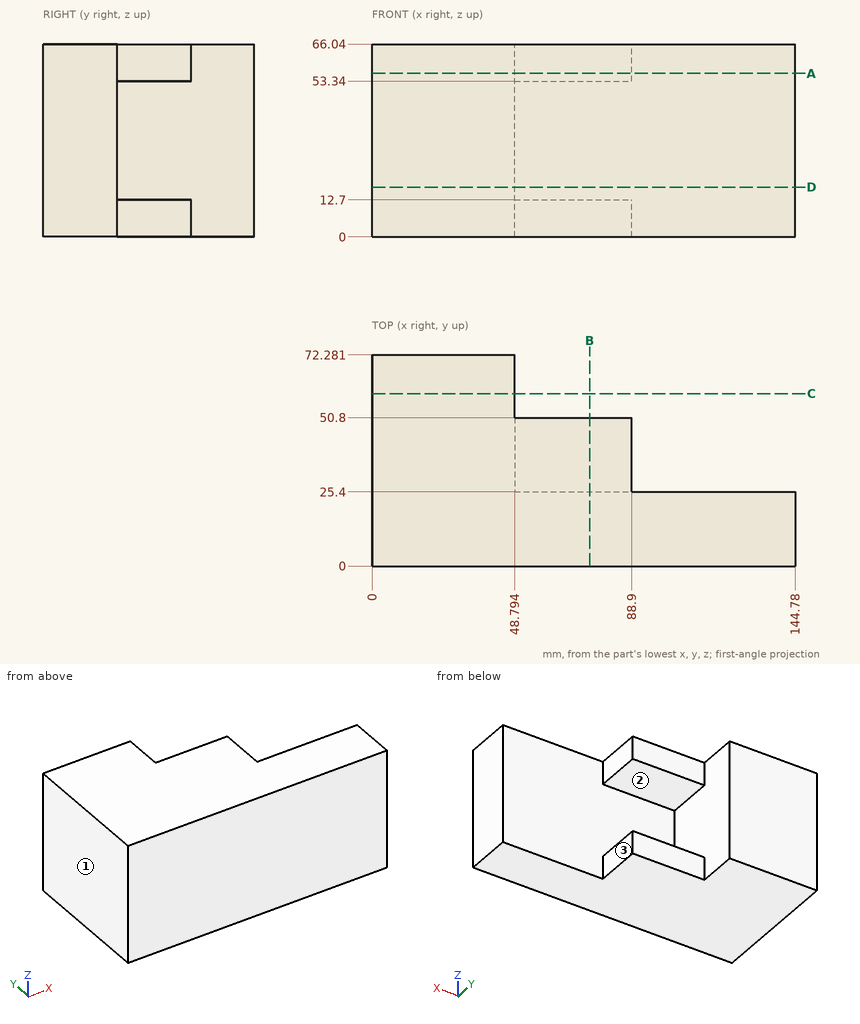
Source: three-view drawing plus pictorial views. Frame: mm from the lowest corner of the part. A direction names the side the tool comes from. Round coordinates to 2 decimals unless told otherwise and drop trailing zeros. Loops run counter-clockwise (first coordinate to the right, second up) from the corner with the lowest first, then second, coordinate; pieces in that order, holes last.
1. Contact query for flat-ended pins moving along their axis: pin 1 (14 mm diameter, centred on x = 76.5, z = 57.5, fed in from +Y); pin 2 (10 mm diameter, centred on y = 36, z = 57, fed in from +X); pin 3 (2 mm diameter, centred on x = 29, y = 35.5, fed in from -Z); pin 4 (4 mm diameter, centred on x = 120, z = 56.5, fed in from +Y). Output: stop coordinate, or through.
2. Access query for the marked faces 1, 2 and 3. Directions: +Z, -Z, +X, -X, +Y, -Y. A direction counts if a zero-diameter tool reaches every point of the face in a straight line with its end or side. Return the directions, or none.
3. Section query A-A on z = 56. Output: boundary loops of the cut face in (x, y).
4. Section query C-C on y = 59. Output: boundary loops of the cut face in (x, z).
5. Ray query, L1, parallel to Z at x = 51, y = 38; L2, parallel to X at y = 44, z = 61; L3, parallel to X at y = 47.5, z = 15.5. Return the intervals inside material, ascending.
6. Section query B-B on x = 74.5. Output: boundary loops of the cut face in (y, z), and give its area (3 significant figures).
7. Section query D-D on z = 17. Output: boundary loops of the cut face in (x, y), and give its area (4 significant figures).
Answers below:
1. pin 1: stops at y = 50.8
1. pin 2: stops at x = 88.9
1. pin 3: stops at z = 0
1. pin 4: stops at y = 25.4
2. face 1: +Z, -Z, -X, +Y, -Y
2. face 2: +X, +Y
2. face 3: +Z, -Z, +X, +Y
3. outline: (0, 0) - (144.78, 0) - (144.78, 25.4) - (88.9, 25.4) - (88.9, 50.8) - (48.79, 50.8) - (48.79, 72.28) - (0, 72.28) - close
4. outline: (0, 0) - (48.79, 0) - (48.79, 66.04) - (0, 66.04) - close
5. L1: z = 0 to 12.7, 53.34 to 66.04
5. L2: x = 0 to 88.9
5. L3: x = 0 to 48.79
6. outline: (0, 0) - (50.8, 0) - (50.8, 12.7) - (25.4, 12.7) - (25.4, 53.34) - (50.8, 53.34) - (50.8, 66.04) - (0, 66.04) - close
6. area: 2,320 mm2
7. outline: (0, 0) - (144.78, 0) - (144.78, 25.4) - (48.79, 25.4) - (48.79, 72.28) - (0, 72.28) - close
7. area: 5,965 mm2
